Can you work these out from the model? Positions are in its coordinate system, mm. Face numbers are marked on the shaded views. A direction names the side the tool comes from. Give positions to 0.01 mm unless a question says otherwise; leave off trailing zeros. Write each loop counter-clockwise with the first axis right and the second up, starting at its lowest first coordinate (ties: lowest second). Pieces come first, ordered by that corner, then holes. Notation, with made-up numbers: M -31,-19.5 L 27,-19.5 A16 cw 27,-12.5 Z; hole C 13,69 d3. An arc over 180 degrees is marked long. Write each question's results on one line, items separated by ' | '.
from build123d import *

# Parameters (mm, degrees)
BRIDA_BASE1_DEPTH     = 19.5
CROQUIS9_R            = 1.5
CORTAR_EXTRUIR4_DEPTH = 0.5
CROQUIS10_R           = 1.5
CORTAR_EXTRUIR5_DEPTH = 0.5


# Sheet-metal steps are written as plain solids
with BuildPart() as part:
    # Croquis1 → Brida base1 (new body)
    with BuildSketch(Plane(origin=(0, 0, 0), x_dir=(0, 0, -1), z_dir=(1, 0, 0))):
        with BuildLine():
            Line((-8.25, 24.950879865), (-0.5, 24.950879865))
            ThreePointArc((-0.5, 24.950879865), (-0.146446609, 24.804433255), (0, 24.450879865))
            Line((0, 24.450879865), (0, 8.950879865))
            Line((0, 8.950879865), (0.5, 8.950879865))
            Line((0.5, 8.950879865), (0.5, 24.450879865))
            ThreePointArc((0.5, 24.450879865), (0.207106781, 25.157986646), (-0.5, 25.450879865))
            Line((-0.5, 25.450879865), (-8.25, 25.450879865))
            Line((-8.25, 25.450879865), (-8.25, 24.950879865))
        make_face()
    extrude(amount=BRIDA_BASE1_DEPTH)

    # Croquis9 → Cortar-Extruir4 (cut)
    with BuildSketch(Plane(origin=(0, 0, -0.5), x_dir=(-1, 0, 0), z_dir=(0, 0, -1))):
        with Locations(Location((-13.75, 17.200879865, 0), (0, 0, 90))):
            Circle(CROQUIS9_R)
        with Locations(Location((-5.75, 17.200879865, 0), (0, 0, 90))):
            Circle(CROQUIS9_R)
    extrude(amount=-CORTAR_EXTRUIR4_DEPTH, mode=Mode.SUBTRACT)

    # Croquis10 → Cortar-Extruir5 (cut)
    with BuildSketch(Plane(origin=(0, 25.450879865, 0), x_dir=(1, 0, 0), z_dir=(0, 1, 0))):
        with Locations(Location((9.75, -4.375, 0), (0, 0, 270))):
            Circle(CROQUIS10_R)
    extrude(amount=-CORTAR_EXTRUIR5_DEPTH, mode=Mode.SUBTRACT)


solid = part.part
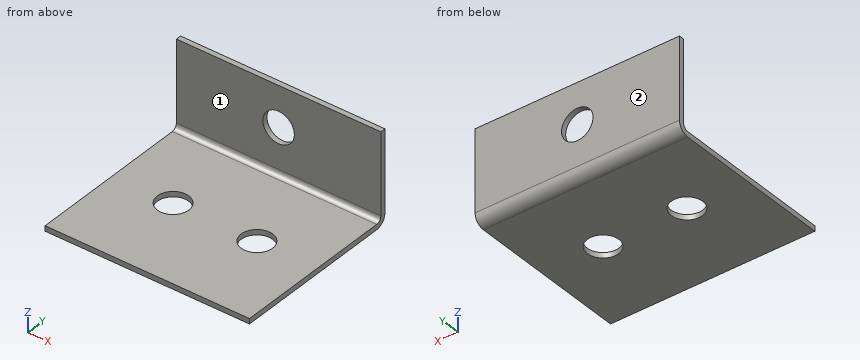
Item 1: I want a section at A-A, the plane x = 9.75. Please give me the cut outline in (y, z) (3 decimals), and give its area (3 significant figures).
Geometry says:
outline: M 8.951,-0.5 L 24.451,-0.5 A1 ccw 25.451,0.5 L 25.451,2.875 L 24.951,2.875 L 24.951,0.5 A0.5 cw 24.451,0 L 8.951,0 Z; M 24.951,5.875 L 25.451,5.875 L 25.451,8.25 L 24.951,8.25 Z | area: 10.7 mm2
Item 2: I want a section at B-B, the plane x = 16.75. Please give me the cut outline in (y, z).
Geometry says:
outline: M 8.95,-0.5 L 24.45,-0.5 A1 ccw 25.45,0.5 L 25.45,8.25 L 24.95,8.25 L 24.95,0.5 A0.5 cw 24.45,0 L 8.95,0 Z
Item 3: If I drill on line 1 (Y direction, x = 12.25, z = 4); line 2 (Z direction, x = 18.5, y = 12.5), over which ranges is the centre line in solid material (lowest first)? Write a range as from..to.
Geometry says:
line 1: y = 24.95..25.45 | line 2: z = -0.5..0
Item 4: I want a section at C-C, the plane z = 1. Please give me the cut outline in (x, y).
Geometry says:
outline: M 0,24.95 L 19.5,24.95 L 19.5,25.45 L 0,25.45 Z
Item 5: For the marked faces 1 and 2, which set-ups out of +Z, -Z, +X, -X, +Y, -Y let a thin tool reach every point of the face, with its end or its side?
Geometry says:
face 1: +Z, +X, -X, -Y | face 2: +Z, -Z, +X, -X, +Y
Item 6: I'm going to push flat-ended pins straight in: pin 1 (4 mm diameter, centred on x = 9.75, z = 4.375, fed in from -Y); pin 2 (6 mm diameter, centred on x = 7, y = 15.5, fed in from +Z). Where does each tip first touch, or does it pass through?
Geometry says:
pin 1: stops at y = 24.95 | pin 2: stops at z = 0
